Model file for the job. Use its own axes, mm. A direction names the side the tool comes from. Give positions to 0.01 mm unless a question says otherwise; leave off trailing zeros. Write each loop counter-clockwise with the first axis right and the second up, starting at its lowest first coordinate (ties: lowest second). Pieces come first, ordered by that corner, then holes. Notation, with made-up numbers: (-39.5, 4) - (10.5, 4) arc R19 cw to (10.5, 29) - close; hole circle Ø9 at (-6, 52). An arc over 180 degrees is marked (long way). Use CSV: the item, a comma, the result in double quotes.
from build123d import *

# Parameters (mm, degrees)
BOSS_EXTRUDE1_START = 16.51
SKETCH2_R           = 6.6675
SKETCH2_R_2         = 47.625
SKETCH2_R_3         = 25.4
BOSS_EXTRUDE1_DEPTH = 16.51
CUT_EXTRUDE1_REACH  = 129.898
SKETCH3_R           = 9.525
CHAMFER1_SIZE       = 0.8128
CHAMFER2_SIZE       = 0.8128
CHAMFER3_SIZE       = 3.175
FILLET2_R           = 1.524


with BuildPart() as part:
    # Sketch1 → Revolve1 (revolve)
    with BuildSketch(Plane.XY, mode=Mode.PRIVATE) as revolve1_sk:
        Polygon((0, 25.4), (53.975, 25.4), (53.975, 47.625), (52.3748, 46.0248), (52.3748, 34.29), (34.925, 34.29), (16.51, 38.204229083), (16.51, 76.2), (1.6002, 76.2), (1.6002, 47.6377), (0, 46.0375), align=None)
    revolve(revolve1_sk.sketch.rotate(Axis((0, 0, 0), (1, 0, 0)), 90), axis=Axis((0, 0, 0), (1, 0, 0)))

    # Sketch2 → Boss-Extrude1 (add)
    # profile 1 of 2: a face of its own
    with BuildSketch(Plane(origin=(53.975, 0, 0), x_dir=(0, 0, -1), z_dir=(1, 0, 0)).offset(BOSS_EXTRUDE1_START)):
        with BuildLine():
            Line((-59.9948, 40.005), (-59.9948, 24.717162721))
            ThreePointArc((-59.9948, 24.717162721), (-60.246417717, 21.150810443), (-60.996285714, 17.655116229))
            ThreePointArc((-60.996285714, 17.655116229), (-63.5, 0), (-60.996285714, -17.655116229))
            ThreePointArc((-60.996285714, -17.655116229), (-60.246417717, -21.150810443), (-59.9948, -24.717162721))
            Line((-59.9948, -24.717162721), (-59.9948, -40.005))
            ThreePointArc((-59.9948, -40.005), (-54.139923135, -54.139923135), (-40.005, -59.9948))
            Line((-40.005, -59.9948), (-24.717162721, -59.9948))
            ThreePointArc((-24.717162721, -59.9948), (-21.150810443, -60.246417717), (-17.655116229, -60.996285714))
            ThreePointArc((-17.655116229, -60.996285714), (0, -63.5), (17.655116229, -60.996285714))
            ThreePointArc((17.655116229, -60.996285714), (21.150810443, -60.246417717), (24.717162721, -59.9948))
            Line((24.717162721, -59.9948), (40.005, -59.9948))
            ThreePointArc((40.005, -59.9948), (54.139923135, -54.139923135), (59.9948, -40.005))
            Line((59.9948, -40.005), (59.9948, -24.717162721))
            ThreePointArc((59.9948, -24.717162721), (60.246417717, -21.150810443), (60.996285714, -17.655116229))
            ThreePointArc((60.996285714, -17.655116229), (63.5, 0), (60.996285714, 17.655116229))
            ThreePointArc((60.996285714, 17.655116229), (60.246417717, 21.150810443), (59.9948, 24.717162721))
            Line((59.9948, 24.717162721), (59.9948, 40.005))
            ThreePointArc((59.9948, 40.005), (54.139923135, 54.139923135), (40.005, 59.9948))
            Line((40.005, 59.9948), (24.717162721, 59.9948))
            ThreePointArc((24.717162721, 59.9948), (21.150810443, 60.246417717), (17.655116229, 60.996285714))
            ThreePointArc((17.655116229, 60.996285714), (0, 63.5), (-17.655116229, 60.996285714))
            ThreePointArc((-17.655116229, 60.996285714), (-21.150810443, 60.246417717), (-24.717162721, 59.9948))
            Line((-24.717162721, 59.9948), (-40.005, 59.9948))
            ThreePointArc((-40.005, 59.9948), (-54.139923135, 54.139923135), (-59.9948, 40.005))
        make_face()
        with Locations((-42.656216575, -42.656216575)):
            Circle(SKETCH2_R, mode=Mode.SUBTRACT)
        with Locations((42.656216575, -42.656216575)):
            Circle(SKETCH2_R, mode=Mode.SUBTRACT)
        with Locations((42.656216575, 42.656216575)):
            Circle(SKETCH2_R, mode=Mode.SUBTRACT)
        with Locations((-42.656216575, 42.656216575)):
            Circle(SKETCH2_R, mode=Mode.SUBTRACT)
        Circle(SKETCH2_R_2, mode=Mode.SUBTRACT)
    # profile 2 of 2: a face of its own
    with BuildSketch(Plane(origin=(53.975, 0, 0), x_dir=(0, 0, -1), z_dir=(1, 0, 0)).offset(BOSS_EXTRUDE1_START)):
        Circle(SKETCH2_R_2)
        with Locations(Location((0, 0, 0), (0, 0, 180))):
            Circle(SKETCH2_R_3, mode=Mode.SUBTRACT)
    extrude(amount=-BOSS_EXTRUDE1_DEPTH)

    # Sketch3 → Cut-Extrude1 (cut, up to next)
    with BuildSketch(Plane.ZY.offset(-1.6002), mode=Mode.PRIVATE) as cut_extrude1_sk1:
        with Locations((-42.656216575, 42.656216575)):
            Circle(SKETCH3_R)
    cut_extrude1_tool1 = extrude(cut_extrude1_sk1.sketch, amount=-CUT_EXTRUDE1_REACH, mode=Mode.PRIVATE) & part.part
    # Sketch3 → Cut-Extrude1 (cut, up to next)
    with BuildSketch(Plane.ZY.offset(-1.6002), mode=Mode.PRIVATE) as cut_extrude1_sk2:
        with Locations((42.656216575, 42.656216575)):
            Circle(SKETCH3_R)
    cut_extrude1_tool2 = extrude(cut_extrude1_sk2.sketch, amount=-CUT_EXTRUDE1_REACH, mode=Mode.PRIVATE) & part.part
    # Sketch3 → Cut-Extrude1 (cut, up to next)
    with BuildSketch(Plane.ZY.offset(-1.6002), mode=Mode.PRIVATE) as cut_extrude1_sk3:
        with Locations((42.656216575, -42.656216575)):
            Circle(SKETCH3_R)
    cut_extrude1_tool3 = extrude(cut_extrude1_sk3.sketch, amount=-CUT_EXTRUDE1_REACH, mode=Mode.PRIVATE) & part.part
    # Sketch3 → Cut-Extrude1 (cut, up to next)
    with BuildSketch(Plane.ZY.offset(-1.6002), mode=Mode.PRIVATE) as cut_extrude1_sk4:
        with Locations((-42.656216575, -42.656216575)):
            Circle(SKETCH3_R)
    cut_extrude1_tool4 = extrude(cut_extrude1_sk4.sketch, amount=-CUT_EXTRUDE1_REACH, mode=Mode.PRIVATE) & part.part
    add(cut_extrude1_tool1.solids().sort_by_distance((1.6002, 42.656217, -42.656217))[0], mode=Mode.SUBTRACT)
    add(cut_extrude1_tool2.solids().sort_by_distance((1.6002, 42.656217, 42.656217))[0], mode=Mode.SUBTRACT)
    add(cut_extrude1_tool3.solids().sort_by_distance((1.6002, -42.656217, 42.656217))[0], mode=Mode.SUBTRACT)
    add(cut_extrude1_tool4.solids().sort_by_distance((1.6002, -42.656217, -42.656217))[0], mode=Mode.SUBTRACT)

    # Chamfer1
    chamfer1_edges = [part.edges().sort_by_distance(p)[0] for p in [
        (70.485, 42.656216575, 49.323716575),
        (70.485, 42.656216575, -35.988716575),
        (70.485, -42.656216575, -35.988716575),
        (70.485, -42.656216575, 49.323716575),
        (53.975, -42.656216575, 49.323716575),
        (53.975, -42.656216575, -35.988716575),
        (53.975, 42.656216575, -35.988716575),
        (53.975, 42.656216575, 49.323716575),
    ]]
    chamfer(chamfer1_edges, length=CHAMFER1_SIZE)

    # Chamfer2
    chamfer2_edges = [part.edges().sort_by_distance(p)[0] for p in [
        (1.6002, -42.656216575, 33.131216575),
        (16.51, -42.656216575, 33.131216575),
        (1.6002, 42.656216575, 33.131216575),
        (16.51, 42.656216575, 33.131216575),
        (1.6002, 42.656216575, -52.181216575),
        (16.51, 42.656216575, -52.181216575),
        (1.6002, -42.656216575, -52.181216575),
        (16.51, -42.656216575, -52.181216575),
    ]]
    chamfer(chamfer2_edges, length=CHAMFER2_SIZE)

    # Chamfer3
    chamfer3_edges = [part.edges().sort_by_distance(p)[0] for p in [
        (0, 0, -25.4),
        (70.485, 0, -25.4),
    ]]
    chamfer(chamfer3_edges, length=CHAMFER3_SIZE)

    # Fillet2
    fillet2_edges = [part.edges().sort_by_distance(p)[0] for p in [
        (16.51, 0, -38.204229083),
        (52.3748, 0, -34.29),
    ]]
    fillet(fillet2_edges, radius=FILLET2_R)


solid = part.part
(1) Flat gauge pins, fed straight in: P1, Ø7.5, axis at x = 62, y = 29, coming from the +Z side; P2, Ø17, axis at x = 66, z = -33.5, coming from the -Y side; P3, Ø8, axis at x = 13.5, y = -45, coming from the +Z side. Where does each tip first touch, or does it go through?
Checked values:
P1,"stops at z = 59.99"
P2,"stops at y = -59.99"
P3,"stops at z = 64.23"
(2) Saw through at C-C, the plane x = 45.5. List the corners of the cut face in (y, z).
Checked values:
outline,"circle Ø68.58 at (0, 0); hole circle Ø50.8 at (0, 0)"
(3) Saw through at D-D, the plane x = 65. Count the separate pieces of the cut face and the enclosed holes in it, then the cut area to 3 significant figures.
Checked values:
separate pieces,"1"
enclosed holes,"5"
area,"11,900 mm^2"
(4) Wall check: probe 1 along X at (y, z) = (15.5, -54.5) (3 decimals); probe 2 along X at (y, z) = (-40, 0.5) (3 decimals); probe 3 along Z at (x, y) = (5, -36.5). Give the ranges that are in metal, low to high. Write a range as [from, to].
Checked values:
probe 1,"x = [1.6, 16.51], [53.975, 70.485]"
probe 2,"x = [0, 16.51], [52.375, 70.485]"
probe 3,"z = [-66.89, -49.92], [-35.39, 35.39], [49.92, 66.89]"
(5) 3-axis set-ups, long thin cutter, end or side, ignore diameter. For faces 4 (the face through (16.51, 33, -33)), 5 (the face through (62, -32, 59.995)), 6 (the face through (62.346, 54.294, 53.984)), 7 (the face through (62.35, 60.24, -21.2)), 8 (the face through (62.334, -36.045, 43.524)): which of +Z, -Z, +X, -X, +Y, -Y reach the whole face in a straight line?
Checked values:
face 4,"none"
face 5,"+Z, +X, -Y"
face 6,"+Z, +X, +Y"
face 7,"-Z, +X, +Y"
face 8,"+X, -X"
(6) Pull direction X, two halves, no side cores. Call faces 1 (the face through (33.85, 33.7, -7.48)), 2 (the face through (62, -32, -59.995)), 3 (the face through (3.021, -7.676, 24.374)): released by +X, released by -X, zero draft, split by the parting line, or undercut.
Checked values:
face 1,"undercut"
face 2,"zero draft"
face 3,"released by -X"
